Design review of the part built by this model. Coordinates are the model's own, in mm. A direction names the side the tool comes from. Round coordinates to 2 decimals unless told otherwise and drop trailing zeros. Order: outer loops, then holes, each group sorted by start corner. A loop starts at its lowest first (then second) coordinate and runs counter-clockwise, first axis right, second up. Notation, with made-up numbers: M 82.5,89 L 117.5,89 A26 ccw 117.5,114 Z; hole C -11.5,-16.75 d1. An arc over 180 degrees is marked long. Use a Markdown table: item, result. Add a question column.
(1) For pin 1 (5 mm diameter, centred on x = 19, z = -15.5, fed in from -Y); pin 2 (5 mm diameter, centred on y = -6, z = -31, fed in from +X), all flat-tipped, find the tip position at first contact; note any pin that passes through.
(2) Take a section at D-D (y = -9). Write out the cut boundary in (x, z).
(3) Take a section at A-A (z = -22). Write out the cut boundary in (x, y).
(4) To check wall thickness, follow probe 1 along Y at (x, z) = (22.25, -22.5); probe 2 along Y at (x, z) = (20, -12); probe 3 along Y at (x, z) = (17.25, -33.25). State the ranges of each line that lie inside material, in increasing order. Write a range as from..to.
(5) Machinability: for faces 1 (the face through (20, -9.8, -25)), 2 (the face through (20, -10, -25)), which of the approach directions +Z, -Z, +X, -X, +Y, -Y give a long, thin tool a straight path to every point of the face, cutting with its end or side? Answer none if there is none.
(6) Take a section at C-C (y = -5). Write out the cut boundary in (x, z).
(7) Take a section at B-B (x = 19.25). Write out the cut boundary in (y, z), then the cut area to 3 significant figures.
```python
from build123d import *

# Parameters (mm, degrees)
SKETCH_1_W = 9.54
SKETCH_1_H = 0.2


with BuildPart() as part:
    # 스윕1: sweep along a path in 스케치3
    with BuildLine(Plane(origin=(20, 0, 0), x_dir=(0, 0, -1), z_dir=(1, 0, 0))) as sweep_1_path:
        Line((8.8, 0), (31.8, 0))
        ThreePointArc((31.8, 0), (36.8, -5), (31.8, -10))
        Line((31.8, -10), (17.9, -10))
    # 스케치1 → 스윕1 (sweep)
    with BuildSketch(Plane(origin=(0, 0, -8.8), x_dir=(-1, 0, 0), z_dir=(0, 0, -1))):
        with Locations((-20, -0.1)):
            Rectangle(SKETCH_1_W, SKETCH_1_H)
    sweep(path=sweep_1_path.line)


solid = part.part
```
Verdict:
| question | item | result |
|---|---|---|
| 1 | pin 1 | stops at y = -10 |
| 1 | pin 2 | passes through |
| 2 | outline | M 15.23,-34.8 L 24.77,-34.8 L 24.77,-34.45 L 15.23,-34.45 Z |
| 3 | outline | M 15.23,-10 L 24.77,-10 L 24.77,-9.8 L 15.23,-9.8 Z; M 15.23,-0.2 L 24.77,-0.2 L 24.77,0 L 15.23,0 Z |
| 4 | probe 1 | y = -10..-9.8, -0.2..0 |
| 4 | probe 2 | y = -0.2..0 |
| 4 | probe 3 | y = -9.79..-9.58, -0.42..-0.21 |
| 5 | face 1 | +Z, +X, -X |
| 5 | face 2 | +Z, -Z, +X, -X, -Y |
| 6 | outline | M 15.23,-36.8 L 24.77,-36.8 L 24.77,-36.6 L 15.23,-36.6 Z |
| 7 | outline | M -10,-31.8 A5 ccw 0,-31.8 L 0,-8.8 L -0.2,-8.8 L -0.2,-31.8 A4.8 cw -9.8,-31.8 L -9.8,-17.9 L -10,-17.9 Z |
| 7 | area | 10.5 mm^2 |
